Here's how the part is built. I have some questions about the finished solid (model axes, mm). A direction names the side the tool comes from. Give positions to 0.01 mm unless a question says otherwise; leave off trailing zeros. Loops run counter-clockwise (first coordinate to the right, second up) from the corner with the lowest first, then second, coordinate; pieces in that order, holes last. Notation, with made-up numbers: (17.25, 16.5) - (56.25, 16.5) arc R14 cw to (56.25, 27.5) - close; hole circle Ø5 at (-22, 78). An arc over 180 degrees is marked (long way). Use a Markdown table: item, result.
from build123d import *

# Parameters (mm, degrees)
T_LE_DE_BASE_PLI_E1_DEPTH                   = 36
FRAISAGE_POUR_VIS_T_TE_FRAIS_E_M31_AT_COUNT = 2
FRAISAGE_POUR_VIS_T_TE_FRAIS_E_M31_AT_PITCH = 16
FRAISAGE_POUR_VIS_T_TE_FRAIS_E_M31_2_COUNT  = 2
FRAISAGE_POUR_VIS_T_TE_FRAIS_E_M31_2_PITCH  = 22.627416998
FRAISAGE_POUR_VIS_T_TE_FRAIS_E_M31_3_COUNT  = 2
FRAISAGE_POUR_VIS_T_TE_FRAIS_E_M31_3_PITCH  = 16
D_GAGEMENT_M41_D                            = 4.5


# Sheet-metal steps are written as plain solids
with BuildPart() as part:
    # Esquisse1 → Tôle de base pliée1 (new body)
    with BuildSketch(Plane(origin=(0, 0, 0), x_dir=(0, 0, -1), z_dir=(1, 0, 0))):
        with BuildLine():
            Line((0, 12.75), (0, 4))
            ThreePointArc((0, 4), (-1.171572875, 1.171572875), (-4, 0))
            Line((-4, 0), (-29, 0))
            Line((-29, 0), (-29, 3))
            Line((-29, 3), (-4, 3))
            ThreePointArc((-4, 3), (-3.292893219, 3.292893219), (-3, 4))
            Line((-3, 4), (-3, 12.75))
            Line((-3, 12.75), (0, 12.75))
        make_face()
    extrude(amount=T_LE_DE_BASE_PLI_E1_DEPTH)

    # Esquisse7 → Fraisage pour vis à tête fraisée M31 (revolve, cut)
    with BuildSketch(Plane(origin=(15.5, 3, 24.5), x_dir=(0, 0, 1), z_dir=(1, 0, 0))):
        Polygon((0, 0), (0, 3), (1.7, 3), (1.7, 1.45), (3.15, 0), align=None)
    fraisage_pour_vis_t_te_frais_e_m31 = revolve(axis=Axis((15.5, 9.35, 24.5), (0, -1, 0)), mode=Mode.SUBTRACT)

    # Fraisage pour vis à tête fraisée M31 at: Fraisage pour vis à tête fraisée M31 ×2
    with Locations(*[(0, 0, -i * FRAISAGE_POUR_VIS_T_TE_FRAIS_E_M31_AT_PITCH) for i in range(1, FRAISAGE_POUR_VIS_T_TE_FRAIS_E_M31_AT_COUNT)]):
        add(fraisage_pour_vis_t_te_frais_e_m31, mode=Mode.SUBTRACT)

    # Fraisage pour vis _ t_te frais_e M31 2: Fraisage pour vis à tête fraisée M31 ×2
    with Locations(*[Vector(0.7071067811865476, 0, -0.7071067811865476) * (i * FRAISAGE_POUR_VIS_T_TE_FRAIS_E_M31_2_PITCH) for i in range(1, FRAISAGE_POUR_VIS_T_TE_FRAIS_E_M31_2_COUNT)]):
        add(fraisage_pour_vis_t_te_frais_e_m31, mode=Mode.SUBTRACT)

    # Fraisage pour vis _ t_te frais_e M31 3: Fraisage pour vis à tête fraisée M31 ×2
    with Locations(*[(i * FRAISAGE_POUR_VIS_T_TE_FRAIS_E_M31_3_PITCH, 0, 0) for i in range(1, FRAISAGE_POUR_VIS_T_TE_FRAIS_E_M31_3_COUNT)]):
        add(fraisage_pour_vis_t_te_frais_e_m31, mode=Mode.SUBTRACT)

    # Dégagement M41 (through all)
    with Locations(Plane.XY.offset(3)):
        with Locations((18, 8.2)):
            Hole(D_GAGEMENT_M41_D / 2)


solid = part.part
(1) If I drill on line 1 (X direction, y = 0.7, z = 8.5); line 2 (Z direction, x = 15.5, y = 1); line 3 (Z direction, x = 15.5, y = 1.05), over which ranges is the centre line in solid material (lowest first)?
A:
| item | result |
|---|---|
| line 1 | 0 to 13.8, 17.2 to 29.8, 33.2 to 36 |
| line 2 | 1.35 to 6.8, 10.2 to 22.8, 26.2 to 29 |
| line 3 | 1.3 to 6.8, 10.2 to 22.8, 26.2 to 29 |
(2) Suppose I cut it at A-A on x = 31.5. Write out the boundary of the cut face in (y, z).
A:
| item | result |
|---|---|
| outline | (0, 4) arc R4 ccw to (4, 0) - (12.75, 0) - (12.75, 3) - (4, 3) arc R1 cw to (3, 4) - (3, 5.35) - (1.55, 6.8) - (0, 6.8) - close; (0, 10.2) - (1.55, 10.2) - (3, 11.65) - (3, 21.35) - (1.55, 22.8) - (0, 22.8) - close; (0, 26.2) - (1.55, 26.2) - (3, 27.65) - (3, 29) - (0, 29) - close |
(3) Will these pins go through, and if not, where does the flat tip stop? pin 1 (2 mm diameter, centred on x = 15.5, z = 24.5, fed in from +Y); pin 2 (4 mm diameter, centred on x = 31.5, z = 8.5, fed in from +Y); pin 3 (6 mm diameter, centred on x = 18, y = 8.2, fed in from +Z); pin 4 (4.5 mm diameter, centred on x = 15.5, z = 8.5, fed in from +Y).
A:
| item | result |
|---|---|
| pin 1 | through |
| pin 2 | y = 1.85 |
| pin 3 | z = 3 |
| pin 4 | y = 2.1 |
(4) We'd pull the mould along Z, two halves only. Please class faces 1 (the face through (17.748, 1.203, 1.141)), 2 (the face through (33, 0.8, 25.3)), 3 (the face through (18, 12.75, 2)): pulls with the +Z half, pulls with the -Z half, needs draft (parallel to the pull), parting line crosses it, or undercut.
A:
| item | result |
|---|---|
| face 1 | pulls with the -Z half |
| face 2 | undercut |
| face 3 | needs draft |
(5) Suppose I cut it at B-B on z = 8.5. Write out the boundary of the cut face in (x, y).
A:
| item | result |
|---|---|
| outline | (0, 0) - (13.8, 0) - (13.8, 1.55) - (12.35, 3) - (0, 3) - close; (17.2, 0) - (29.8, 0) - (29.8, 1.55) - (28.35, 3) - (18.65, 3) - (17.2, 1.55) - close; (33.2, 0) - (36, 0) - (36, 3) - (34.65, 3) - (33.2, 1.55) - close |
(6) On a 3-axis mill with a long thin cutter (end or side, diameter ignored), from which of +Z, -Z, +X, -X, +Y, -Y can I reach the whole of each face in a straight line? I mean faces 4 (the face through (18, 11, 3)), 5 (the face through (30.067, 0.786, 9.414)). Say none if no direction works.
A:
| item | result |
|---|---|
| face 4 | +Z, +X, -X, +Y |
| face 5 | +Y, -Y |
(7) Suppose I cut it at D-D on x = 2.5. Write out the boundary of the cut face in (y, z).
A:
| item | result |
|---|---|
| outline | (0, 4) arc R4 ccw to (4, 0) - (12.75, 0) - (12.75, 3) - (4, 3) arc R1 cw to (3, 4) - (3, 29) - (0, 29) - close |
(8) Suppose I cut it at C-C on y = 8.2. Write out the boundary of the cut face in (x, z), plus the area to 3 significant figures.
A:
| item | result |
|---|---|
| outline | (0, 0) - (15.75, 0) - (15.75, 3) - (0, 3) - close; (20.25, 0) - (36, 0) - (36, 3) - (20.25, 3) - close |
| area | 94.5 mm2 |
